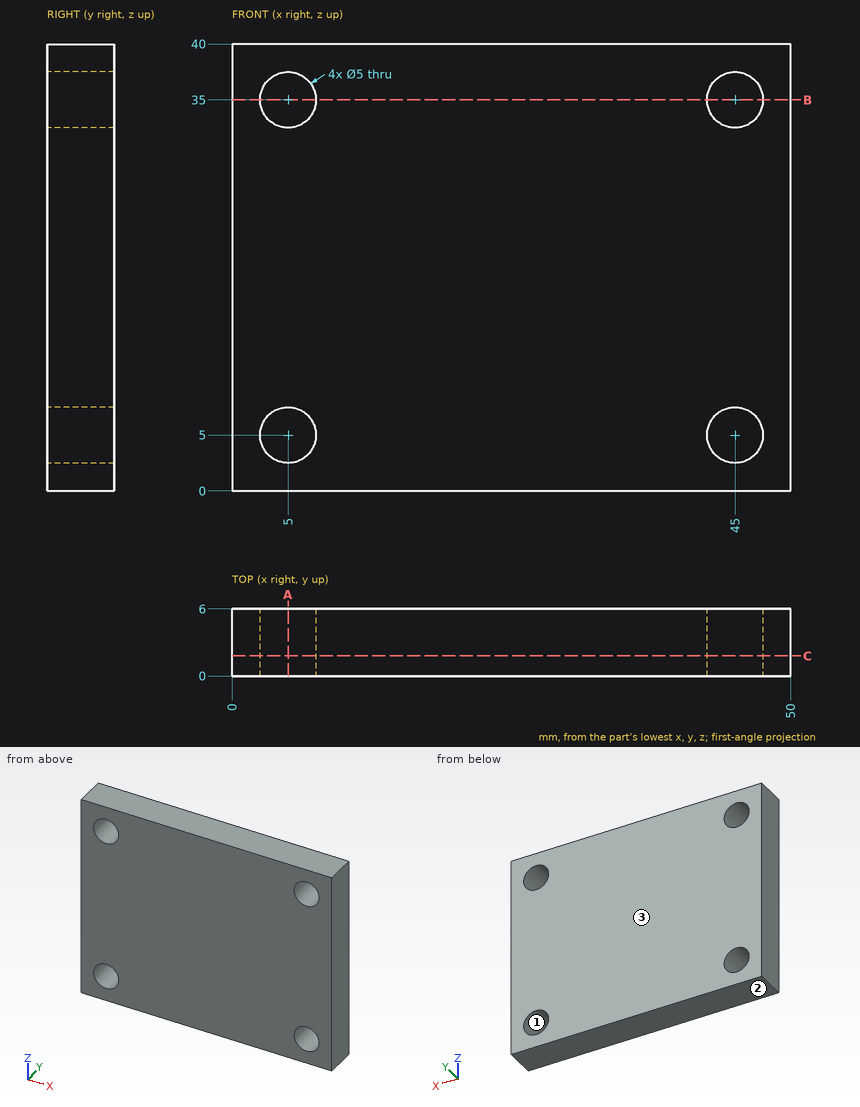
Geometry check sheet. Reference: drawing and pictorial views, mm from the part's lowest x, y, z. Round coordinates to 2 decimals unless told otherwise and drop trailing zeros. Order: outer loops, then holes, each group sorted by start corner. A loop starts at its lowest first (then second) coordinate and runs counter-clockwise, first axis right, second up. Notation, with made-up numbers: M 69,41.5 L 103,41.5 A13 cw 103,49.5 Z; hole C 79.25,78 d2. An arc over 180 degrees is marked long. Answer in a Markdown table with one row per item.
(1) Sectioned sample at A-A, the plane x = 5. Record the cut outline in (y, z), and give its area (3 significant figures).
Responses:
| item | result |
|---|---|
| outline | M 0,0 L 6,0 L 6,2.5 L 0,2.5 Z; M 0,7.5 L 6,7.5 L 6,32.5 L 0,32.5 Z; M 0,37.5 L 6,37.5 L 6,40 L 0,40 Z |
| area | 180 mm² |
(2) Sectioned sample at C-C, the plane y = 1.8. Record the cut outline in (x, z), and give its area (3 significant figures).
Responses:
| item | result |
|---|---|
| outline | M 0,0 L 50,0 L 50,40 L 0,40 Z; hole C 5,5 d5; hole C 5,35 d5; hole C 45,5 d5; hole C 45,35 d5 |
| area | 1,920 mm² |
(3) Sectioned sample at B-B, the plane z = 35. Record the cut outline in (x, y).
Responses:
| item | result |
|---|---|
| outline | M 0,0 L 2.5,0 L 2.5,6 L 0,6 Z; M 7.5,0 L 42.5,0 L 42.5,6 L 7.5,6 Z; M 47.5,0 L 50,0 L 50,6 L 47.5,6 Z |
(4) Scan lines: probe 1 along Z at (x, y) = (5, 2.4); probe 2 along Z at (x, y) = (6, 0.35); probe 3 along X at (y, z) = (0.3, 4.5). Record each from-to range of solid material in increasing order. Write a range as from..to.
Responses:
| item | result |
|---|---|
| probe 1 | z = 0..2.5, 7.5..32.5, 37.5..40 |
| probe 2 | z = 0..2.71, 7.29..32.71, 37.29..40 |
| probe 3 | x = 0..2.55, 7.45..42.55, 47.45..50 |
(5) Draft check along Z on the marked faces 1, 2 and 3. Enter one of: released by +Z, released by -Z, zero draft, split by the parting line, or undercut.
Responses:
| item | result |
|---|---|
| face 1 | undercut |
| face 2 | released by -Z |
| face 3 | zero draft |
